CAD build for the part. Positions are in the model's coordinates, mm. A direction names the side the tool comes from. Coordinates: 2 decimals unless noted, no trailing zeros. Loops run counter-clockwise (first coordinate to the right, second up) from the corner with the lowest first, then second, coordinate; pieces in that order, holes last. Notation, with made-up numbers: (-12.75, -10) -> (39.25, -10) arc R20 ccw to (39.25, 29) -> close; hole circle Ø4 at (-29.5, -32). An arc over 180 degrees is marked (long way). Answer as a JSON object with one key per item and string values. Group by question number.
from build123d import *

# Parameters (mm, degrees)
SKETCH1_R           = 12
BOSS_EXTRUDE1_DEPTH = 2
SKETCH2_R           = 19
BOSS_EXTRUDE2_DEPTH = 5
FILLET1_R           = 2
SKETCH3_R           = 6
SKETCH3_R_2         = 1.4
CUT_EXTRUDE1_DEPTH  = 28.766886822


with BuildPart() as part:
    # Sketch1 → Boss-Extrude1 (new body)
    with BuildSketch(Plane(origin=(0, 0, 0), x_dir=(1, 0, 0), z_dir=(0, 1, 0))):
        with Locations(Location((0, 0, 0), (0, 0, 270))):
            Circle(SKETCH1_R)
    extrude(amount=BOSS_EXTRUDE1_DEPTH)

    # Sketch2 → Boss-Extrude2 (add)
    with BuildSketch(Plane(origin=(0, 2, 0), x_dir=(1, 0, 0), z_dir=(0, 1, 0))):
        with Locations(Location((0, 0, 0), (0, 0, 270))):
            Circle(SKETCH2_R)
    extrude(amount=BOSS_EXTRUDE2_DEPTH)

    # Fillet1
    fillet1_edges = [part.edges().sort_by_distance(p)[0] for p in [
        (0, 7, -19),
    ]]
    fillet(fillet1_edges, radius=FILLET1_R)

    # Sketch3 → Cut-Extrude1 (cut, through all)
    with BuildSketch(Plane(origin=(0, 7, 0), x_dir=(1, 0, 0), z_dir=(0, 1, 0))):
        with Locations(Location((0, 0, 0), (0, 0, 270))):
            Circle(SKETCH3_R)
        with Locations(Location((0, 15, 0), (0, 0, 270))):
            Circle(SKETCH3_R_2)
        with Locations(Location((12.990381057, 7.5, 0), (0, 0, 270))):
            Circle(SKETCH3_R_2)
        with Locations(Location((12.990381057, -7.5, 0), (0, 0, 270))):
            Circle(SKETCH3_R_2)
        with Locations(Location((0, -15, 0), (0, 0, 270))):
            Circle(SKETCH3_R_2)
        with Locations(Location((-12.990381057, -7.5, 0), (0, 0, 270))):
            Circle(SKETCH3_R_2)
        with Locations(Location((-12.990381057, 7.5, 0), (0, 0, 270))):
            Circle(SKETCH3_R_2)
    extrude(amount=-CUT_EXTRUDE1_DEPTH, mode=Mode.SUBTRACT)


solid = part.part
Item 1: Band-saw the part on B-B, the plane x = 0. List the corners of the cut face in (y, z).
Item 2: Band-saw the part on C-C, the plane y = 3.75. List the corners of the cut face in (x, z), and give its area (3 significant figures).
Item 3: Pull direction X, two halves, no side cores. Call faces 3 (the flat face through (0, 7, 7)), 4 (the cylindrical face through (13.94, 4.54, 6.47)), 5 (the cylindrical face through (-11.56, 3.48, -15.08)), 6 (the cylindrical face through (13.94, 4.54, -8.53)): +X half, -X half, draft (parallel to the pull), parting line (faces both ways), or undercut.
Item 4: Band-saw the part on D-D, the plane y = 1.25. List the corners of the cut face in (x, z).
Item 5: 3-axis set-ups, long thin cutter, end or side, ignore diameter. For faces 1 (the cylindrical face through (-14.357, 4.535, -7.803)), 2 (the cylindrical face through (3.604, 0.986, 11.446)): which of +Z, -Z, +X, -X, +Y, -Y reach the whole face in a straight line?
Item 6: Band-saw the part on A-A, the plane z = 0. List the corners of the cut face in (x, y).
Item 7: Flat gauge pins, fed straight in: P1, Ø1.5, axis at y = 1, z = -7.5, coming from the +X side; P2, Ø1, axis at x = 8, y = 5, coming from the -Z side; P3, Ø4, axis at x = -5.5, y = 2.5, coming from the +Z side. Where does each tip first touch, or does it go through?
Item 8: Drill centre lines: L1, parallel to X at y = 5, z = -7.5; L2, parallel to Z at x = 1, y = 6; L3, parallel to X at y = 6.5, z = 7.5. Where is each one in solid material? Low to high.
Reply:
{
 "1": {"outline": "(0, -12) -> (2, -12) -> (2, -13.6) -> (7, -13.6) -> (7, -6) -> (0, -6) -> close; (0, 6) -> (7, 6) -> (7, 13.6) -> (2, 13.6) -> (2, 12) -> (0, 12) -> close; (2, -19) -> (5, -19) arc R2 ccw to (7, -17) -> (7, -16.4) -> (2, -16.4) -> close; (2, 16.4) -> (7, 16.4) -> (7, 17) arc R2 ccw to (5, 19) -> (2, 19) -> close"},
 "2": {"outline": "circle Ø38 at (0, 0); hole circle Ø2.8 at (-12.99, -7.5); hole circle Ø2.8 at (-12.99, 7.5); hole circle Ø12 at (0, 0); hole circle Ø2.8 at (0, -15); hole circle Ø2.8 at (0, 15); hole circle Ø2.8 at (12.99, -7.5); hole circle Ø2.8 at (12.99, 7.5)", "area": "984 mm²"},
 "3": {"face 3": "draft", "face 4": "undercut", "face 5": "parting line", "face 6": "undercut"},
 "4": {"outline": "circle Ø24 at (0, 0); hole circle Ø12 at (0, 0)"},
 "5": {"face 1": "+Y, -Y", "face 2": "-Y"},
 "6": {"outline": "(-19, 2) -> (-12, 2) -> (-12, 0) -> (-6, 0) -> (-6, 7) -> (-17, 7) arc R2 ccw to (-19, 5) -> close; (6, 0) -> (12, 0) -> (12, 2) -> (19, 2) -> (19, 5) arc R2 ccw to (17, 7) -> (6, 7) -> close"},
 "7": {"P1": "x = 9.92", "P2": "z = -17.46", "P3": "z = 18.67"},
 "8": {"L1": "-17.46 to -14.39, -11.59 to 11.59, 14.39 to 17.46", "L2": "-18.71 to -15.98, -14.02 to -5.92, 5.92 to 14.02, 15.98 to 18.71", "L3": "-16.72 to -14.39, -11.59 to 11.59, 14.39 to 16.72"}
}
